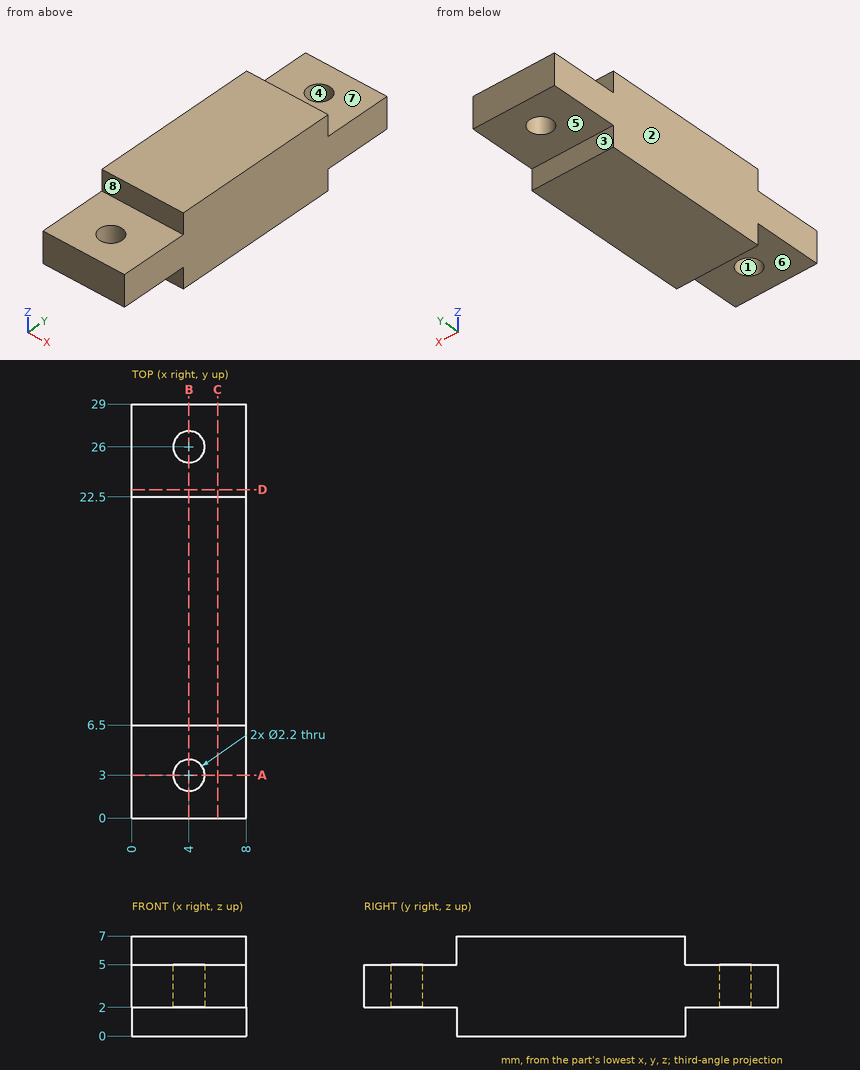
Study the drawing (mm; zero at the part's minimum x, y, z) and answer. A direction names the side the tool comes from. Round coordinates to 2 decimals unless told otherwise and drop trailing zeros. Loops run counter-clockwise (first coordinate to the right, second up) from the corner with the lowest first, then second, coordinate; pieces in that order, holes last. Notation, with made-up numbers: (6.25, 1.5) - (58.25, 1.5) arc R27 ccw to (58.25, 21.5) - close; hole circle Ø5 at (85, 24.5). An arc over 180 degrees is marked (long way). Use one line per item in the form item = value. Start each with the question number.
1. The part is cut by section A-A on y = 3. Determine the outline of the cut face in (x, z).
2. For a pull along X with two mould halves and no side action, classify the marked faces 1, 2 and 3 as pulls with the +X half, pulls with the -X half, needs draft (parallel to the pull), parting line crosses it, or undercut.
3. Given pin 1 Ø1 at (x, z) = (6, 1) entering from +Y; pin 2 Ø0.6 at (x, z) = (4, 1) entering from -Y; pin 3 Ø3 at (x, y) = (6, 3) entering from -Z, each flat-ended and moving along its own axis, determine where each tip first touches the part or whether it passes through.
4. The part is cut by section C-C on x = 6. Determine the outline of the cut face in (y, z).
5. Consider line 1 (Y direction, x = 4, z = 2.6); line 2 (Y direction, x = 5, z = 2.75); line 3 (Y direction, x = 3, z = 1.5). Determine where each line is inside the solid, lowest interval first. Write a range as [from, to].
6. The part is cut by section B-B on x = 4. Determine the outline of the cut face in (y, z), then the cut area to 3 significant figures.
7. The part is cut by section D-D on y = 23. Determine the outline of the cut face in (x, z).
8. A tool of negligible diameter and unlimited length cuts with its end or side. For the marked faces 4, 5, 6, 7 and 8, from which of +Z, -Z, +X, -X, +Y, -Y can it reach the whole face along a straight path? Write none if from no direction.
Geometry check:
q1.outline = (0, 2) - (2.9, 2) - (2.9, 5) - (0, 5) - close; (5.1, 2) - (8, 2) - (8, 5) - (5.1, 5) - close
q2.face_1 = undercut
q2.face_2 = pulls with the -X half
q2.face_3 = needs draft
q3.pin_1 = 22.5
q3.pin_2 = 6.5
q3.pin_3 = 2
q4.outline = (0, 2) - (6.5, 2) - (6.5, 0) - (22.5, 0) - (22.5, 2) - (29, 2) - (29, 5) - (22.5, 5) - (22.5, 7) - (6.5, 7) - (6.5, 5) - (0, 5) - close
q5.line_1 = [0, 1.9], [4.1, 24.9], [27.1, 29]
q5.line_2 = [0, 2.54], [3.46, 25.54], [26.46, 29]
q5.line_3 = [6.5, 22.5]
q6.outline = (0, 2) - (1.9, 2) - (1.9, 5) - (0, 5) - close; (4.1, 2) - (6.5, 2) - (6.5, 0) - (22.5, 0) - (22.5, 2) - (24.9, 2) - (24.9, 5) - (22.5, 5) - (22.5, 7) - (6.5, 7) - (6.5, 5) - (4.1, 5) - close; (27.1, 2) - (29, 2) - (29, 5) - (27.1, 5) - close
q6.area = 138 mm^2
q7.outline = (0, 2) - (8, 2) - (8, 5) - (0, 5) - close
q8.face_4 = +Z, -Z
q8.face_5 = -Z, +X, -X, +Y
q8.face_6 = -Z, +X, -X, -Y
q8.face_7 = +Z, +X, -X, +Y
q8.face_8 = +Z, +X, -X, -Y
